```python
from build123d import *


with BuildPart() as f1:
    # F0 (on Front) → F1 (revolve)
    with BuildSketch(Plane.XZ):
        with BuildLine():
            ThreePointArc((-91.44, 58.42), (-98.918451, 49.459225), (-101.6, 38.1))
            Line((-101.6, 38.1), (-101.6, -38.1))
            ThreePointArc((-101.6, -38.1), (-98.918451, -49.459225), (-91.44, -58.42))
            Line((-91.44, -58.42), (-33.02, -102.235))
            Line((-33.02, -102.235), (0, -102.235))
            Line((0, -102.235), (0, 102.235))
            Line((0, 102.235), (-33.02, 102.235))
            Line((-33.02, 102.235), (-91.44, 58.42))
        make_face()
    revolve(axis=Axis((0, 0, 4.563034), (0, 0, -1)))


solid = f1.part
```
Model file for the job. Use its own axes, mm. Give positions to 0.01 mm unless a question says otherwise; leave off trailing zeros. Loops run counter-clockwise (first coordinate to the right, second up) from the corner with the lowest first, then second, coordinate; pieces in that order, holes last. Notation, with made-up numbers: M -15,26.25 L -6,26.25 A31 ccw -6,62.25 Z; hole C 3.25,40.5 d11. An arc over 180 degrees is marked long. Use one line per item in the form item = value.
Item 1: Flat gauge pins, fed straight in: pin 1 Ø12 at (y, z) = (-74.5, -3) entering from +X; pin 2 Ø2 at (x, y) = (-12, 77.5) entering from -Z; pin 3 Ø1.5 at (x, y) = (40, 15.5) entering from -Z. Where does each tip first touch, or does it go through?
Filled in:
pin_1 = 75.04
pin_2 = -68.93
pin_3 = -95.39
Item 2: Drill centre lines: L1, parallel to Y at x = -30, z = -93.5; L2, parallel to X at y = 9.5, z = 50.5; L3, parallel to X at y = 47.5, z = -21.5. Where is each one in solid material? Low to high.
Filled in:
L1 = -33.09 to 33.09
L2 = -97.91 to 97.91
L3 = -89.81 to 89.81
Item 3: Slice it at C-C on z = 67. List the corners of the cut face in (x, y), and give its area (3 significant figures).
Filled in:
outline = C 0,0 d160
area = 20,100 mm^2
Item 4: Slice it at A-A on x = 0. List the corners of the cut face in (y, z) (3 decimals), and give its area (3 significant figures).
Filled in:
outline = M -101.6,-38.1 A25.4 ccw -91.44,-58.42 L -33.02,-102.235 L 33.02,-102.235 L 91.44,-58.42 A25.4 ccw 101.6,-38.1 L 101.6,38.1 A25.4 ccw 91.44,58.42 L 33.02,102.235 L -33.02,102.235 L -91.44,58.42 A25.4 ccw -101.6,38.1 Z
area = 34,400 mm^2
